```python
from build123d import *

# Parameters (mm, degrees)
F0_W          = 118
F0_H          = 180
F1_DEPTH      = 63
F2_W          = 116
F2_H          = 179
F3_DEPTH      = 62.5
F5_DEPTH      = 88
F5_DEPTH_BACK = 88
F6_SIZE2      = 2.0997279246
F6_SIZE       = 24
F6_2_SIZE2    = 2.0997279246
F6_2_SIZE     = 24
F7_R          = 5
F8_W          = 48
F8_H          = 2.5
F9_DEPTH      = 2
F11_DEPTH     = 1


with BuildPart() as f1:
    # F0 (on Top) → F1 (new body)
    with BuildSketch(Plane.XY):
        Rectangle(F0_W, F0_H)
    extrude(amount=F1_DEPTH)

    # F2 (on face) → F3 (cut)
    with BuildSketch(Plane.XY.offset(63)):
        Rectangle(F2_W, F2_H)
    extrude(amount=-F3_DEPTH, mode=Mode.SUBTRACT)

    # F4 (on Front) → F5 (join, two sides)
    with BuildSketch(Plane.XZ) as f5_sk:
        Polygon((-142.0850467894, 146.0850467894), (-59, 63), (-57.9865276814, 63), (-141.2585024524, 146.271974771), (-134.8901262921, 170.0390781628), (-135.6145706619, 170.2331924466), align=None)
    extrude(amount=F5_DEPTH)
    extrude(f5_sk.sketch, amount=-F5_DEPTH_BACK)

    # F6
    f6_edges = [f1.edges().sort_by_distance(p)[0] for p in [
        (-135.252348, -88, 170.136135),
    ]]
    f6_side = f1.faces().sort_by_distance((-100.446161, -88, 104.638886))[0]
    chamfer(f6_edges, length=F6_SIZE, length2=F6_SIZE2, reference=f6_side)

    # F6#2
    f6_2_edges = [f1.edges().sort_by_distance(p)[0] for p in [
        (-135.252348, 88, 170.136135),
    ]]
    f6_2_side = f1.faces().sort_by_distance((-100.446161, 88, 104.638886))[0]
    chamfer(f6_2_edges, length=F6_2_SIZE, length2=F6_2_SIZE2, reference=f6_2_side)

    # F7
    f7_edges = [f1.edges().sort_by_distance(p)[0] for p in [
        (-135.252348, 85.900272, 170.136135),
        (-135.252348, -85.900272, 170.136135),
    ]]
    fillet(f7_edges, radius=F7_R)

    # F8 (on face) → F9 (cut)
    with BuildSketch(Plane(origin=(0, 90, 0), x_dir=(-1, 0, 0), z_dir=(0, 1, 0))):
        with Locations((0, 31.5)):
            Rectangle(F8_W, F8_H)
    extrude(amount=-F9_DEPTH, mode=Mode.SUBTRACT)

    # F10 (on face) → F11 (join)
    with BuildSketch(Plane(origin=(2.5067361593, 0, 2.5067361593), x_dir=(0.7071067812, 0, -0.7071067812), z_dir=(0.7071067812, 0, 0.7071067812))):
        with BuildLine():
            Line((-202.3147502425, -86.6807101745), (-86.5503941557, -86.6807101745))
            Line((-86.5503941557, -86.6807101745), (-86.5503941557, 66.6807101745))
            Line((-86.5503941557, 66.6807101745), (-124.3079604016, 66.6807101745))
            ThreePointArc((-124.3079604016, 66.6807101745), (-127.8936462296, 65.4914125289), (-130.0578494866, 62.3949958888))
            ThreePointArc((-130.0578494866, 62.3949958888), (-144.4325721991, 51.6807101745), (-158.8072949116, 62.3949958888))
            ThreePointArc((-158.8072949116, 62.3949958888), (-160.9714981686, 65.4914125289), (-164.5571839966, 66.6807101745))
            Line((-164.5571839966, 66.6807101745), (-202.3147502425, 66.6807101745))
            Line((-202.3147502425, 66.6807101745), (-202.3147502425, -86.6807101745))
        make_face()
    extrude(amount=F11_DEPTH)


solid = f1.part
```
Part model, mm, in its own coordinate system. A direction names the side the tool comes from. Coordinates: 2 decimals unless noted, no trailing zeros. Order: outer loops, then holes, each group sorted by start corner. A loop starts at its lowest first (then second) coordinate and runs counter-clockwise, first axis right, second up. Notation, with made-up numbers: (-13, -5.75) - (15, -5.75) arc R13 ccw to (15, 6.25) - close; hole circle Ø1 at (-11, -28.75). An arc over 180 degrees is marked (long way). Return JSON: item names as keys, results as strings. Group by question number.
Item 1: Drill centre lines: probe 1 along Y at (x, z) = (-10, 23.5); probe 2 along X at (y, z) = (24, 27); probe 3 along Z at (x, y) = (-52.5, 14). Where is each one in solid material? Low to high. Write a range as from..to.
Item 2: Pin check, flat tips, straight feed: pin 1 (3 mm diameter, centred on y = -32, z = 131.5, fed in from -X); pin 2 (19 mm diameter, centred on y = -42, z = 21, fed in from -X); pin 3 (0.6 mm diameter, centred on x = 7.5, y = 90, fed in from +Z). Stop position of each tip, or through.
Item 3: Which spindle directions (+Z, -Z, +X, -X, +Y, -Y) get a long thin tool onto all of the face, cutting with end or side? Do faces 5 (the face through (-1, -89.5, 32)), 6 (the face through (59, -1, 31)), 7 (the face through (-71.5, 66.681, 77.2)), 8 (the face through (-138.805, -1.232, 158.328)), 9 (the face through (-59, -1, 31)). Say none if no direction does.
Item 4: Cut at B-B (z = 27.5). List the corners of the cut face in (x, y).
Item 5: Cut at C-C (x = -49.5). List the corners of the cut face in (y, z).
Item 6: Cut at A-A (x = 3.5). List the corners of the cut face in (y, z), plus the area to 3 significant figures.
Item 7: Pull direction Z, two halves, no side cores. Call faces 1 (the face through (-138.12, -1.23, 157.99)), 2 (the face through (-1, 1, 0.5)), 3 (the face through (-101, -1, 105)), 4 (the face through (-58, -1, 32)): pulls with the +Z half, pulls with the -Z half, needs draft (parallel to the pull), parting line crosses it, or undercut.
Check values:
{
 "1": {"probe 1": "y = -90..-89.5, 89.5..90", "probe 2": "x = -59..-58, 58..59", "probe 3": "z = 0..0.5"},
 "2": {"pin 1": "stops at x = -129", "pin 2": "stops at x = -59", "pin 3": "stops at z = 63"},
 "3": {"face 5": "+Z", "face 6": "+Z, -Z, +X, +Y, -Y", "face 7": "+Z, +X, +Y", "face 8": "+Z, -X, +Y, -Y", "face 9": "-Z, -X, +Y, -Y"},
 "4": {"outline": "(-59, -90) - (59, -90) - (59, 90) - (-59, 90) - close; hole (-58, -89.5) - (58, -89.5) - (58, 89.5) - (-58, 89.5) - close"},
 "5": {"outline": "(-90, 0) - (90, 0) - (90, 63) - (89.5, 63) - (89.5, 0.5) - (-89.5, 0.5) - (-89.5, 63) - (-90, 63) - close"},
 "6": {"outline": "(-90, 0) - (90, 0) - (90, 30.25) - (89.5, 30.25) - (89.5, 0.5) - (-89.5, 0.5) - (-89.5, 63) - (-90, 63) - close; (89.5, 32.75) - (90, 32.75) - (90, 63) - (89.5, 63) - close", "area": "151 mm2"},
 "7": {"face 1": "undercut", "face 2": "pulls with the +Z half", "face 3": "pulls with the -Z half", "face 4": "needs draft"}
}
